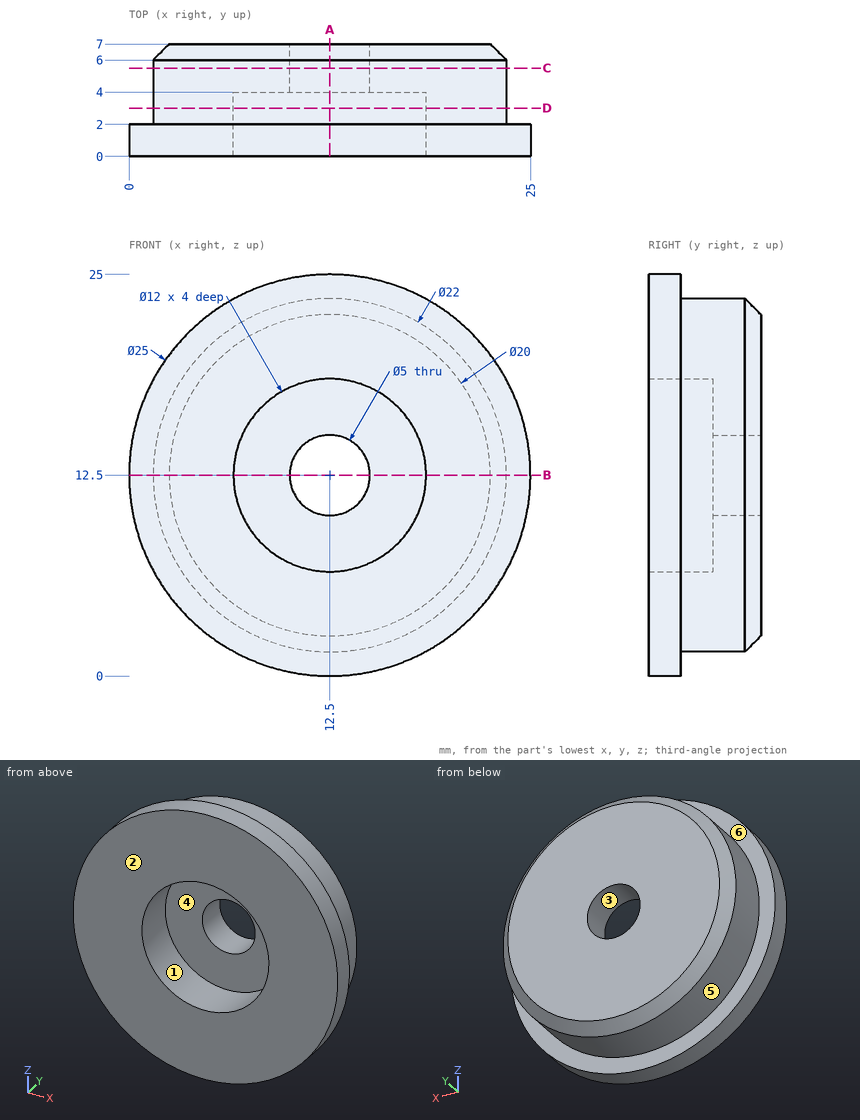
Here's the drawing with two shaded views (mm, measured from the low corner). I have some questions. A direction names the side the tool comes from. Round coordinates to 2 decimals unless told otherwise and drop trailing zeros. Loops run counter-clockwise (first coordinate to the right, second up) from the corner with the lowest first, then second, coordinate; pieces in that order, holes last. Notation, with made-up numbers: (68, 88) - (91, 88) arc R29 cw to (91, 110) - close; hole circle Ø2 at (8, 70). An arc over 180 degrees is marked (long way). Use CSV: the item, a comma, the result in double quotes.
Item 1: I need wall thicknesses on L1, parallel to Z at x = 12.5, y = 3.15; L2, parallel to Z at x = 12.5, y = 1.6. Which ranges of each line are inside material? Lowest first, please. Write a range as [from, to].
Here are the results:
L1,"z = [1.5, 6.5], [18.5, 23.5]"
L2,"z = [0, 6.5], [18.5, 25]"
Item 2: For the marked faces 1 and 2, which set-ups out of +Z, -Z, +X, -X, +Y, -Y let a thin tool reach every point of the face, with its end or its side?
Here are the results:
face 1,"-Y"
face 2,"+Z, -Z, +X, -X, -Y"
Item 3: If we section it at A-A on x = 12.5: List the corners of the cut face in (y, z) for me.
Here are the results:
outline,"(0, 0) - (2, 0) - (2, 1.5) - (6, 1.5) - (7, 2.5) - (7, 10) - (4, 10) - (4, 6.5) - (0, 6.5) - close; (0, 18.5) - (4, 18.5) - (4, 15) - (7, 15) - (7, 22.5) - (6, 23.5) - (2, 23.5) - (2, 25) - (0, 25) - close"
Item 4: Will these pins go through, and if not, where does the flat tip stop? pin 1 (2 mm diameter, centred on y = 5, z = 11, fed in from +X); pin 2 (1.5 mm diameter, centred on x = 7.5, y = 1.5, fed in from -Z); pin 3 (3.5 mm diameter, centred on x = 10.5, z = 15, fed in from -Y).
Here are the results:
pin 1,"stops at x = 23.49"
pin 2,"stops at z = 0.74"
pin 3,"stops at y = 4"
Item 5: If we section it at C-C on y = 5.5: List the corners of the cut face in (x, z) for me, then the cut area to 3 significant figures.
Here are the results:
outline,"circle Ø22 at (12.5, 12.5); hole circle Ø5 at (12.5, 12.5)"
area,"360 mm²"
Item 6: If we section it at B-B on z = 12.5: List the corners of the cut face in (x, y) for me, then the cut area to 3 significant figures.
Here are the results:
outline,"(0, 0) - (6.5, 0) - (6.5, 4) - (10, 4) - (10, 7) - (2.5, 7) - (1.5, 6) - (1.5, 2) - (0, 2) - close; (15, 4) - (18.5, 4) - (18.5, 0) - (25, 0) - (25, 2) - (23.5, 2) - (23.5, 6) - (22.5, 7) - (15, 7) - close"
area,"96.0 mm²"
Item 7: If we mould it in two halves opening along X, with no side actions, what happens to the marked faces 3, 4, 5 and 6? For each: pulls with the +X half, pulls with the -X half, needs draft (parallel to the pull), parting line crosses it, or undercut.
Here are the results:
face 3,"undercut"
face 4,"undercut"
face 5,"parting line crosses it"
face 6,"needs draft"
Item 8: If we section it at D-D on y = 3: List the corners of the cut face in (x, z) for me, then the cut area to 3 significant figures.
Here are the results:
outline,"circle Ø22 at (12.5, 12.5); hole circle Ø12 at (12.5, 12.5)"
area,"267 mm²"
